Model file for the job. Use its own axes, mm. A direction names the side the tool comes from. Round coordinates to 2 decimals unless told otherwise and drop trailing zeros. Loops run counter-clockwise (first coordinate to the right, second up) from the corner with the lowest first, then second, coordinate; pieces in that order, holes last. Notation, with made-up numbers: (33.5, 85) - (89.5, 85) arc R31 ccw to (89.5, 123) - close; hole circle Ø10 at (20.25, 69). An arc over 180 degrees is marked (long way). Use one line per item in the form item = value.
from build123d import *

# Parameters (mm, degrees)
SKETCH1_R           = 2.5
BOSS_EXTRUDE1_DEPTH = 2


with BuildPart() as part:
    # Sketch1 → Boss-Extrude1 (new, symmetric)
    with BuildSketch(Plane(origin=(0, 0, 0), x_dir=(1, 0, 0), z_dir=(0, 1, 0))):
        with BuildLine():
            Line((-25.876894374, 4), (25.876894374, 4))
            ThreePointArc((25.876894374, 4), (26.819703416, 4.112698737), (27.709385764, 4.444444444))
            ThreePointArc((27.709385764, 4.444444444), (35, 0), (27.709385764, -4.444444444))
            ThreePointArc((27.709385764, -4.444444444), (26.819703416, -4.112698737), (25.876894374, -4))
            Line((25.876894374, -4), (-25.876894374, -4))
            ThreePointArc((-25.876894374, -4), (-26.819703416, -4.112698737), (-27.709385764, -4.444444444))
            ThreePointArc((-27.709385764, -4.444444444), (-35, 0), (-27.709385764, 4.444444444))
            ThreePointArc((-27.709385764, 4.444444444), (-26.819703416, 4.112698737), (-25.876894374, 4))
        make_face()
        with Locations(Location((-30, 0, 0), (0, 0, 270))):
            Circle(SKETCH1_R, mode=Mode.SUBTRACT)
        with Locations(Location((30, 0, 0), (0, 0, 270))):
            Circle(SKETCH1_R, mode=Mode.SUBTRACT)
    extrude(amount=BOSS_EXTRUDE1_DEPTH, both=True)


solid = part.part
1. Tool access for faces 1 (the cylindrical face through (-26.81, 0.03, 4.11)), 2 (the cylindrical face through (-35, 0, 0)), 3 (the flat face through (0, 0, -4)): list every direction of +Z, -Z, +X, -X, +Y, -Y with a clear straight run to the whole face (end or side of a thin tool).
Geometry check:
face_1 = +Z, +Y, -Y
face_2 = +Y, -Y
face_3 = -Z, +Y, -Y
2. Cut at B-B, the plane x = -30. Give the cut face in (y, z).
Geometry check:
outline = (-2, -5) - (2, -5) - (2, -2.5) - (-2, -2.5) - close; (-2, 2.5) - (2, 2.5) - (2, 5) - (-2, 5) - close
3. Cut at A-A, the plane z = 0. Give the cut face in (x, y).
Geometry check:
outline = (-35, -2) - (-32.5, -2) - (-32.5, 2) - (-35, 2) - close; (-27.5, -2) - (27.5, -2) - (27.5, 2) - (-27.5, 2) - close; (32.5, -2) - (35, -2) - (35, 2) - (32.5, 2) - close
4. Flat gauge pins, fed straight in: pin 1 (1 mm diameter, centred on x = 24.5, y = 0, fed in from +Z); pin 2 (2 mm diameter, centred on x = -13, y = -1, fed in from -Z). Where does each tip first touch, or does it go through?
Geometry check:
pin_1 = 4
pin_2 = -4
5. Cut at C-C, the plane y = 0.65. Give the cut face in (x, z).
Geometry check:
outline = (-27.71, -4.44) arc R4 cw to (-25.88, -4) - (25.88, -4) arc R4 cw to (27.71, -4.44) arc R5 ccw (long way) to (27.71, 4.44) arc R4 cw to (25.88, 4) - (-25.88, 4) arc R4 cw to (-27.71, 4.44) arc R5 ccw (long way) to start; hole circle Ø5 at (-30, 0); hole circle Ø5 at (30, 0)
6. Pull direction Z, two halves, no side cores. Call faces 4 (the cylindrical face through (-27.52, -0.03, -0.33)), 5 (the flat face through (0, -2, 0)), 6 (the flat face through (0, 0, 4)): +Z half, -Z half, draft (parallel to the pull), parting line (faces both ways), or undercut.
Geometry check:
face_4 = undercut
face_5 = draft
face_6 = +Z half
7. Wall check: probe 1 along X at (y, z) = (0.6, 0); probe 2 along X at (y, z) = (-0.85, -1); probe 3 along Z at (x, y) = (-15, -1.55). Give the ranges that are in metal, low to high.
Geometry check:
probe_1 = -35 to -32.5, -27.5 to 27.5, 32.5 to 35
probe_2 = -34.9 to -32.29, -27.71 to 27.71, 32.29 to 34.9
probe_3 = -4 to 4
8. Cut at D-D, the plane x = -22.5. Give the cut face in (y, z).
Geometry check:
outline = (-2, -4) - (2, -4) - (2, 4) - (-2, 4) - close
